Model file for the job. Use its own axes, mm. A direction names the side the tool comes from. Give positions to 0.01 mm unless a question says otherwise; leave off trailing zeros. Loops run counter-clockwise (first coordinate to the right, second up) from the corner with the lowest first, then second, coordinate; pieces in that order, holes last. Notation, with made-up numbers: (77, 53.25) -> (130, 53.25) arc R26 cw to (130, 68.25) -> close; hole circle Ø1 at (0, -21). An arc over 180 degrees is marked (long way). Use CSV: the item, a comma, the result in double quotes. Start each with the question number.
(1) Cut at A-A on x = 0. Write the cut outline in (y, z), then the cut area to 3 significant figures.
(2) Cut at B-B on y = -2. Write the cut outline in (x, z), then the cut area to 3 significant figures.
(3) Drill centre lines: probe 1 along Y at (x, z) = (0, 0.25); probe 2 along Y at (x, z) = (0.5, 1.5); probe 3 along Z at (x, y) = (0.5, -0.5). Where is each one in solid material? Low to high.
(4) Flat gauge pins, fed straight in: pin 1 (3 mm diameter, centred on x = -2, y = -8, fed in from -Z); pin 2 (2 mm diameter, centred on x = -2, z = -2, fed in from -Y); pin 3 (1 mm diameter, centred on x = -0.5, y = -5, fed in from -Z). Where does each tip first touch, or does it go through?
(5) Pull direction Z, two halves, no side cores. Call faces 3 (the flat face through (0, -0.5, -1)), 4 (the flat face through (1.2, -1, 1.2)), 5 (the flat face through (-0.87, -0.49, 0.49)), 6 (the cylindrical face through (-0.45, -4.9, 1.43)): pulls with the +Z half, pulls with the -Z half, needs draft (parallel to the pull), parting line crosses it, or undercut.
(6) 3-axis set-ups, long thin cutter, end or side, ignore diameter. For faces 1 (the flat face through (0, -9, 0)), 2 (the flat face through (0, -1, 0)): which of +Z, -Z, +X, -X, +Y, -Y reach the whole face in a straight line?
from build123d import *

# Parameters (mm, degrees)
CHAMFER_1_SIZE      = 0.3
CUT_EXTRUDE_1_DEPTH = 1


with BuildPart() as part:
    # 草图1 → 旋转1 (revolve)
    with BuildSketch(Plane.XY, mode=Mode.PRIVATE) as revolve_1_sk:
        with BuildLine():
            Line((0, 0), (2.866025404, 0))
            ThreePointArc((2.866025404, 0), (3, -0.5), (2.866025404, -1))
            Line((2.866025404, -1), (1.5, -1))
            Line((1.5, -1), (1.5, -9))
            Line((1.5, -9), (0, -9))
            Line((0, -9), (0, 0))
        make_face()
    revolve(revolve_1_sk.sketch.rotate(Axis((0, 0, 0), (0, -1, 0)), 90), axis=Axis((0, 0, 0), (0, -1, 0)))

    # 倒角1
    chamfer_1_edges = [part.edges().sort_by_distance(p)[0] for p in [
        (0, -9, -1.5),
    ]]
    chamfer(chamfer_1_edges, length=CHAMFER_1_SIZE)

    # 草图2 → 切除-拉伸1 (cut)
    with BuildSketch(Plane(origin=(0, 0, 0), x_dir=(1, 0, 0), z_dir=(0, 1, 0))):
        Polygon((1.154700538, 0), (0.577350269, 1), (-0.577350269, 1), (-1.154700538, 0), (-0.577350269, -1), (0.577350269, -1), align=None)
    extrude(amount=-CUT_EXTRUDE_1_DEPTH, mode=Mode.SUBTRACT)


solid = part.part
Check result:
1,outline,"(-9, -1.2) -> (-8.7, -1.5) -> (-1, -1.5) -> (-1, -2.87) arc R1 ccw to (0, -2.87) -> (0, -1) -> (-1, -1) -> (-1, 1) -> (0, 1) -> (0, 2.87) arc R1 ccw to (-1, 2.87) -> (-1, 1.5) -> (-8.7, 1.5) -> (-9, 1.2) -> close"
1,area,"27.8 mm²"
2,outline,"circle Ø3 at (0, 0)"
2,area,"7.07 mm²"
3,probe 1,"-9 to -1"
3,probe 2,"-1 to 0"
3,probe 3,"-2.96 to -1, 1 to 2.96"
4,pin 1,"z = -1.41"
4,pin 2,"y = -1"
4,pin 3,"z = -1.5"
5,face 3,"undercut"
5,face 4,"needs draft"
5,face 5,"undercut"
5,face 6,"parting line crosses it"
6,face 1,"+Z, -Z, +X, -X, -Y"
6,face 2,"+Y"
